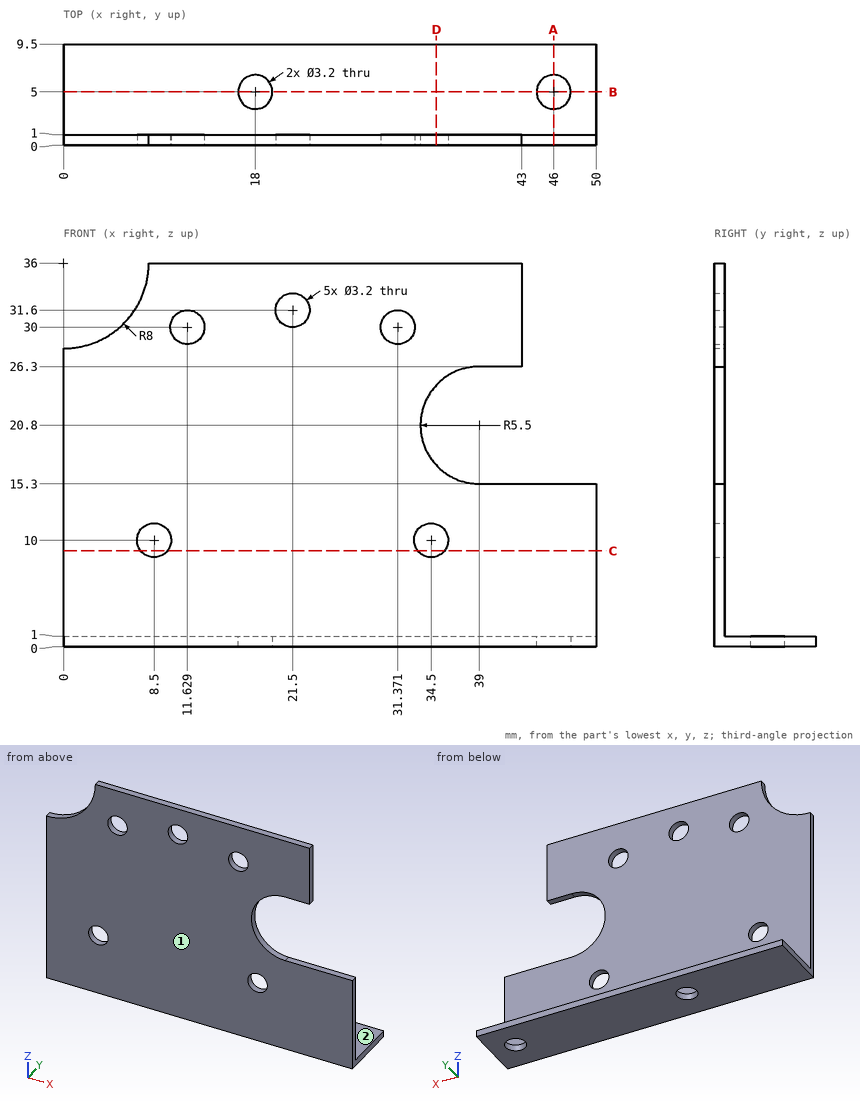
Geometry check sheet. Reference: drawing and pictorial views, mm from the part's lowest x, y, z. A direction names the side the tool comes from. Round coordinates to 2 decimals unless told otherwise and drop trailing zeros. Order: outer loops, then holes, each group sorted by start corner. A loop starts at its lowest first (then second) coordinate and runs counter-clockwise, first axis right, second up. Notation, with made-up numbers: (88.25, 86) - (138.25, 86) arc R15 ccw to (138.25, 109) - close; hole circle Ø9 at (40, 36). An arc over 180 degrees is marked (long way). Use a Markdown table: item, result. Add a question column.
1) Section check B-B (y = 5). Record the cut outline in (x, z), then the cut area to 3 significant figures.
2) Gauge pin test, flat ends, axial feed: P1, Ø3, axis at x = 34.5, z = 10, coming from the -Y side; P2, Ø6, axis at x = 12, z = 32, coming from the +Y side; P3, Ø0.5, axis at x = 44, y = 0.5, coming from the +Z side; P4, Ø1, axis at x = 20.5, y = 6, coming from the +Z side. Record the tip position at first contact, or that the pin passes through.
3) Set-up check for the marked faces 1 and 2: record each of +Z, -Z, +X, -X, +Y, -Y from which the full face is reachable in a straight line by a thin tool's end or side.
4) Thickness scan on line 1 along X through (y, z) = (0.4, 10); line 2 along Y through (x, z) = (46, 0.65); line 3 along Z through (x, y) = (34.5, 0.2). Record the ranges inside material, lowest first.
5) Section check A-A (x = 46). Record the cut outline in (y, z), then the cut area to 3 significant figures.
6) Section check C-C (z = 9). Record the cut outline in (x, y).
7) Section check D-D (x = 35). Record the cut outline in (y, z) (3 decimals), then the cut area to 3 significant figures.
Established:
| question | item | result |
|---|---|---|
| 1 | outline | (0, 0) - (16.4, 0) - (16.4, 1) - (0, 1) - close; (19.6, 0) - (44.4, 0) - (44.4, 1) - (19.6, 1) - close; (47.6, 0) - (50, 0) - (50, 1) - (47.6, 1) - close |
| 1 | area | 43.6 mm2 |
| 2 | P1 | through |
| 2 | P2 | y = 1 |
| 2 | P3 | z = 15.3 |
| 2 | P4 | z = 1 |
| 3 | face 1 | +Z, -Z, +X, -X, -Y |
| 3 | face 2 | +Z, +X, -X, +Y |
| 4 | line 1 | 0 to 6.9, 10.1 to 32.9, 36.1 to 50 |
| 4 | line 2 | 0 to 3.4, 6.6 to 9.5 |
| 4 | line 3 | 0 to 8.4, 11.6 to 17.64, 23.96 to 36 |
| 5 | outline | (0, 0) - (3.4, 0) - (3.4, 1) - (1, 1) - (1, 15.3) - (0, 15.3) - close; (6.6, 0) - (9.5, 0) - (9.5, 1) - (6.6, 1) - close |
| 5 | area | 20.6 mm2 |
| 6 | outline | (0, 0) - (7.25, 0) - (7.25, 1) - (0, 1) - close; (9.75, 0) - (33.25, 0) - (33.25, 1) - (9.75, 1) - close; (35.75, 0) - (50, 0) - (50, 1) - (35.75, 1) - close |
| 7 | outline | (0, 0) - (9.5, 0) - (9.5, 1) - (1, 1) - (1, 8.48) - (0, 8.48) - close; (0, 11.52) - (1, 11.52) - (1, 17.025) - (0, 17.025) - close; (0, 24.575) - (1, 24.575) - (1, 36) - (0, 36) - close |
| 7 | area | 33.9 mm2 |
